Design review of the part built by this model. Coordinates are the model's own, in mm. Coordinates: 2 decimals unless noted, no trailing zeros. Loops run counter-clockwise (first coordinate to the right, second up) from the corner with the lowest first, then second, coordinate; pieces in that order, holes last. Notation, with made-up numbers: (-3.5, -30.5) -> (38.5, -30.5) arc R21 cw to (38.5, -10.5) -> close; hole circle Ø11 at (51, 67.5). An arc over 180 degrees is marked (long way). Answer in a Markdown table with one row per item.
```python
from build123d import *

# Parameters (mm, degrees)
SKETCH1_R           = 45
BOSS_EXTRUDE1_DEPTH = 422.470348
SKETCH2_R           = 13.873885303
CUT_EXTRUDE1_DEPTH  = 428.236696621
CHAMFER1_SIZE       = 4.644584


with BuildPart() as part:
    # Sketch1 → Boss-Extrude1 (new body)
    with BuildSketch(Plane(origin=(0, 0, 0), x_dir=(1, 0, 0), z_dir=(0, 1, 0))):
        with Locations(Location((0, 0, 0), (0, 0, 270))):
            Circle(SKETCH1_R)
    extrude(amount=BOSS_EXTRUDE1_DEPTH)

    # Sketch2 → Cut-Extrude1 (cut, through all)
    with BuildSketch(Plane(origin=(0, 0, 0), x_dir=(1, 0, 0), z_dir=(0, 1, 0))):
        with Locations(Location((0, 0, 0), (0, 0, 270))):
            Circle(SKETCH2_R)
    extrude(amount=CUT_EXTRUDE1_DEPTH, mode=Mode.SUBTRACT)

    # Chamfer1
    chamfer1_edges = [part.edges().sort_by_distance(p)[0] for p in [
        (0, 0, -45),
        (0, 422.470348, -45),
    ]]
    chamfer(chamfer1_edges, length=CHAMFER1_SIZE)


solid = part.part
```
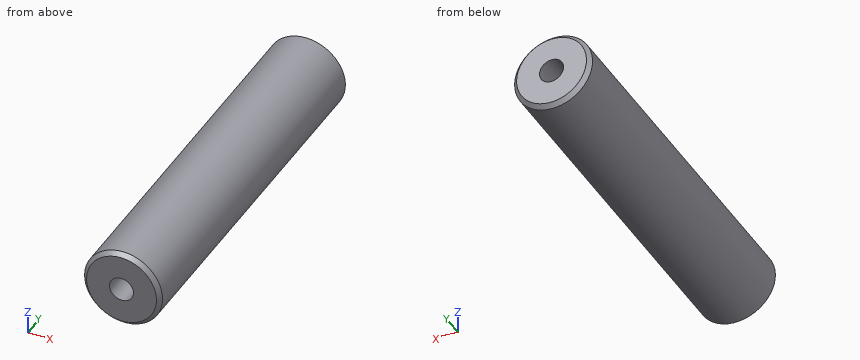
(1) Take a section at A-A on x = 0. Give the boundary of the cut face in (y, z), and give its area (3 significant figures).
Evaluation:
| item | result |
|---|---|
| outline | (0, -40.36) -> (4.64, -45) -> (417.83, -45) -> (422.47, -40.36) -> (422.47, -13.87) -> (0, -13.87) -> close; (0, 13.87) -> (422.47, 13.87) -> (422.47, 40.36) -> (417.83, 45) -> (4.64, 45) -> (0, 40.36) -> close |
| area | 26,300 mm² |
(2) Take a section at B-B on z = 0. Give the boundary of the cut face in (x, y).
Evaluation:
| item | result |
|---|---|
| outline | (-45, 4.64) -> (-40.36, 0) -> (-13.87, 0) -> (-13.87, 422.47) -> (-40.36, 422.47) -> (-45, 417.83) -> close; (13.87, 0) -> (40.36, 0) -> (45, 4.64) -> (45, 417.83) -> (40.36, 422.47) -> (13.87, 422.47) -> close |
(3) Take a section at C-C on y = 70.5. Give the boundary of the cut face in (x, z).
Evaluation:
| item | result |
|---|---|
| outline | circle Ø90 at (0, 0); hole circle Ø27.75 at (0, 0) |
(4) For pin 1 (6 mm diameter, centred on y = 197.5, z = 5, fed in from -X); pin 2 (3 mm diameter, centred on x = 22.5, y = 72.5, fed in from +Z); pin 3 (12 mm diameter, centred on x = -15, y = 377, fed in from +Z), all flat-tipped, find the tip position at first contact; note any pin that passes through.
Evaluation:
| item | result |
|---|---|
| pin 1 | stops at x = -44.96 |
| pin 2 | stops at z = 39.8 |
| pin 3 | stops at z = 44.09 |
(5) To check wall thickness, follow probe 1 along X at (y, z) = (122, 0); probe 2 along X at (y, z) = (136.5, 9.5); probe 3 along Z at (x, y) = (-6, 160.5). State the ranges of each line that lie inside material, in increasing order.
Evaluation:
| item | result |
|---|---|
| probe 1 | x = -45 to -13.87, 13.87 to 45 |
| probe 2 | x = -43.99 to -10.11, 10.11 to 43.99 |
| probe 3 | z = -44.6 to -12.51, 12.51 to 44.6 |
